Geometry: final body of the model. Coordinates: model frame, mm. A direction names the side the tool comes from. Coordinates: 2 decimals unless noted, no trailing zeros. Write each loop counter-clockwise with the first axis right and the second up, starting at its lowest first coordinate (ties: lowest second). Pieces come first, ordered by that corner, then holes. Notation, with made-up numbers: M 76,46 L 81,46 A30 cw 81,81 Z; hole C 83.25,6.5 d7. An arc over 180 degrees is marked long. Write item = value, one per line. Start each with the question number.
Item 1: Reachability of faces 1 (the flat face through (5, 76.2, 32)), 2 (the flat face through (110, 0, 32)) from +Z, -Z, +X, -X, +Y, -Y: full face, straight path, thin tool, end or side. Return the list, or none.
Item 2: Section B-B on y = 29. Output: boundary loops of the cut face in (x, z), plus the area to 3 significant figures.
Item 3: Section C-C on x = 92. Output: boundary loops of the cut face in (y, z), plus the area to 3 significant figures.
Item 4: First-contact query: pin 1 Ø12 at (x, z) = (81.5, 46.5) entering from +Y; pin 2 Ø1 at (y, z) = (2.5, 49.5) entering from +X. Flat tips, straight axial feed; report the tip coordinate or a pass-through.
Item 5: Ray query, L1, parallel to Y at x = 136, z = 16; L2, parallel to X at y = 62, z = 40. Return the intervals inside material, ascending. Write a range as [from, to].
Item 6: Section A-A on z = 13. Output: boundary loops of the cut face in (x, y).
from build123d import *

# Parameters (mm, degrees)
F0_W      = 34.599658
F0_H      = 65.455198
F1_DEPTH  = 50.8
F1_FACE_W = 50.8
F1_FACE_H = 65.455198
F2_DEPTH  = 152.4
F3_DEPTH  = 76.2
F3_FACE_W = 127
F3_FACE_H = 65.455198
F4_DEPTH  = 25.4


with BuildPart() as f1:
    # F0 (on Front) → F1 (new body)
    with BuildSketch(Plane.XZ):
        with Locations((17.299829, 32.727599)):
            Rectangle(F0_W, F0_H)
    extrude(amount=F1_DEPTH)

    # F1_face (on face) → F2 (join)
    with BuildSketch(Plane(origin=(34.599658, -25.4, 32.727599), x_dir=(0, 1, 0), z_dir=(1, 0, 0))):
        Rectangle(F1_FACE_W, F1_FACE_H)
    extrude(amount=F2_DEPTH)

    # F0 (on Front) → F3 (join)
    with BuildSketch(Plane.XZ):
        with Locations((17.299829, 32.727599)):
            Rectangle(F0_W, F0_H)
    extrude(amount=-F3_DEPTH)

    # F3_face (on face) → F4 (join)
    with BuildSketch(Plane(origin=(0, 12.7, 32.727599), x_dir=(0, -1, 0), z_dir=(-1, 0, 0))):
        Rectangle(F3_FACE_W, F3_FACE_H)
    extrude(amount=F4_DEPTH)


solid = f1.part
Responses:
q1.face_1 = +Z, -Z, +X, -X, +Y
q1.face_2 = +Z, -Z, +X, +Y
q2.outline = M -25.4,0 L 34.6,0 L 34.6,65.46 L -25.4,65.46 Z
q2.area = 3,930 mm²
q3.outline = M -50.8,0 L 0,0 L 0,65.46 L -50.8,65.46 Z
q3.area = 3,330 mm²
q4.pin_1 = 0
q4.pin_2 = 34.6
q5.L1 = [-50.8, 0]
q5.L2 = [-25.4, 34.6]
q6.outline = M -25.4,-50.8 L 187,-50.8 L 187,0 L 34.6,0 L 34.6,76.2 L -25.4,76.2 Z
